Could you check a few things on this model? Use its own coordinates, in mm. A direction names the side the tool comes from. Coordinates: 2 decimals unless noted, no trailing zeros. Loops run counter-clockwise (first coordinate to the right, second up) from the corner with the lowest first, then second, coordinate; pieces in that order, holes last.
from build123d import *

# Parameters (mm, degrees)
SKIZZE2_R                       = 1.825
SKIZZE2_R_2                     = 2.9
AUFSATZ_LINEAR_AUSTRAGEN1_DEPTH = 10
SCHNITT_LINEAR_START            = -2.75
SCHNITT_LINEAR_AUSTRAGEN1_DEPTH = 2.75
VERRUNDUNG1_R                   = 10
VERRUNDUNG2_R                   = 10
AUFSATZ_LINEAR_START            = -7.25
SKIZZE5_R                       = 9
SKIZZE5_R_2                     = 5
AUFSATZ_LINEAR_AUSTRAGEN2_DEPTH = 7.25
AUFSATZ_LINEAR_AUSTRAGEN3_DEPTH = 7.25
KREISMUSTER1_COUNT              = 20
SCHNITT_LINEAR_AUSTRAGEN3_DEPTH = 39.948684188


with BuildPart() as part:
    # Skizze2 → Aufsatz-Linear austragen1 (new body)
    with BuildSketch(Plane(origin=(0, 0, 0), x_dir=(1, 0, 0), z_dir=(0, 1, 0))):
        with BuildLine():
            Line((-25, 5), (25, 5))
            ThreePointArc((25, 5), (30, 0), (25, -5))
            Line((25, -5), (-25, -5))
            ThreePointArc((-25, -5), (-30, 0), (-25, 5))
        make_face()
        with Locations(Location((-25, 0, 0), (0, 0, 270))):
            Circle(SKIZZE2_R, mode=Mode.SUBTRACT)
        with Locations(Location((25, 0, 0), (0, 0, 270))):
            Circle(SKIZZE2_R_2, mode=Mode.SUBTRACT)
    extrude(amount=AUFSATZ_LINEAR_AUSTRAGEN1_DEPTH)

    # Skizze4 → Schnitt-Linear austragen1 (cut)
    with BuildSketch(Plane(origin=(0, 10, 0), x_dir=(1, 0, 0), z_dir=(0, 1, 0)).offset(SCHNITT_LINEAR_START)):
        with BuildLine():
            Line((25, 5), (0, 5))
            Line((0, 5), (0, -5))
            Line((0, -5), (25, -5))
            ThreePointArc((25, -5), (30, 0), (25, 5))
        make_face()
    extrude(amount=SCHNITT_LINEAR_AUSTRAGEN1_DEPTH, mode=Mode.SUBTRACT)

    # Verrundung1
    # the kernel refuses this fillet: 10 mm, written as the material it adds along each edge
    with BuildSketch(Plane(origin=(0, 7.25, -5), x_dir=(1, 0, 0), z_dir=(0, 0, 1))) as verrundung1_piece_1:
        with BuildLine():
            CenterArc((6.887488657, 10), VERRUNDUNG1_R, 226.468847833, 43.531152167)
            Line((0, 2.75), (-0.137749773, 2.605))
            ThreePointArc((-0.137749773, 2.605), (-0.2, 1.375), (-0.2, 0))
            Line((-0.2, 0), (0, -0.2))
            Line((0, -0.2), (6.887488657, -0.2))
            Line((6.887488657, -0.2), (6.887488657, 0))
        make_face()
    extrude(amount=10)

    # Verrundung2
    verrundung2_edges = [part.edges().sort_by_distance(p)[0] for p in [
        (0, 10, 0),
    ]]
    fillet(verrundung2_edges, radius=VERRUNDUNG2_R)

    # Skizze5 → Aufsatz-Linear austragen2 (add)
    with BuildSketch(Plane(origin=(0, 7.25, 0), x_dir=(1, 0, 0), z_dir=(0, 1, 0)).offset(AUFSATZ_LINEAR_START)):
        with Locations((25, 0)):
            Circle(SKIZZE5_R)
        with Locations((25, 0)):
            Circle(SKIZZE5_R_2, mode=Mode.SUBTRACT)
    extrude(amount=AUFSATZ_LINEAR_AUSTRAGEN2_DEPTH)

    # Skizze6 → Aufsatz-Linear austragen3 (add)
    with BuildSketch(Plane(origin=(0, 7.25, 0), x_dir=(1, 0, 0), z_dir=(0, 1, 0)).offset(AUFSATZ_LINEAR_START)):
        with BuildLine():
            Line((36, -0.35), (36, 0.35))
            ThreePointArc((36, 0.35), (34.995800842, 0.693259833), (33.954886934, 0.9))
            ThreePointArc((33.954886934, 0.9), (34, 0), (33.954886934, -0.9))
            ThreePointArc((33.954886934, -0.9), (34.995800842, -0.693259833), (36, -0.35))
        make_face()
    aufsatz_linear_austragen3 = extrude(amount=AUFSATZ_LINEAR_AUSTRAGEN3_DEPTH)

    # Kreismuster1: Aufsatz-Linear austragen3 ×20 about axis
    kreismuster1_axis = Axis((25, 0, 0), (0, 1, 0))
    for i in range(1, KREISMUSTER1_COUNT):
        add(aufsatz_linear_austragen3.rotate(kreismuster1_axis, i * 360 / KREISMUSTER1_COUNT))

    # Skizze9 → Schnitt-Linear austragen3 (cut, through all)
    with BuildSketch(Plane.XZ):
        with BuildLine():
            Line((-11, 3), (11, 3))
            ThreePointArc((11, 3), (14, 0), (11, -3))
            Line((11, -3), (-11, -3))
            ThreePointArc((-11, -3), (-14, 0), (-11, 3))
        make_face()
    extrude(amount=-SCHNITT_LINEAR_AUSTRAGEN3_DEPTH, mode=Mode.SUBTRACT)


solid = part.part
(1) I need wall thicknesses on probe 1 along X at (y, z) = (3, 0) (3 decimals); probe 2 along Z at (x, y) = (-6, 2.5); probe 3 along Z at (x, y) = (25, 2.75). Which ranges of each line are inside material? Lowest first, please.
Answers:
probe 1: x = -30 to -26.825, -23.175 to -14, 14 to 22.1, 27.9 to 36
probe 2: z = -5 to -3, 3 to 5
probe 3: z = -11 to -2.9, 2.9 to 11
(2) Imagine slicing it at B-B, the plane x = -13. Write out the boundary of the cut face in (y, z), and give its area (3 significant figures).
Answers:
outline: (0, -5) - (10, -5) - (10, -2.24) - (0, -2.24) - close; (0, 2.24) - (10, 2.24) - (10, 5) - (0, 5) - close
area: 55.3 mm2
(3) Imagine slicing it at D-D, the plane x = 13. Write out the boundary of the cut face in (y, z).
Answers:
outline: (0, -5) - (7.25, -5) - (7.25, -2.24) - (0, -2.24) - close; (0, 2.24) - (7.25, 2.24) - (7.25, 5) - (0, 5) - close
(4) Imagine slicing it at C-C, the plane y = 5.5. State how many separate pieces and enclosed holes the cut face has, and give its area (3 significant figures).
Answers:
separate pieces: 1
enclosed holes: 3
area: 557 mm2
(5) For pin 1 (2 mm diameter, centred on y = 6, z = -7, fed in from +X); pin 2 (2 mm diameter, centred on y = 4.5, z = -4.5, fed in from -X); pin 3 (3 mm diameter, centred on x = 9.5, y = 8.5, fed in from +Z); pin 4 (3.5 mm diameter, centred on x = 25, z = 0, fed in from +Y), each with a flat end and sliding along its axis, tell me the tip position at first contact or that it passes through.
Answers:
pin 1: stops at x = 34.1
pin 2: stops at x = -28.57
pin 3: stops at z = 5
pin 4: passes through
(6) We'd pull the mould along X, two halves only. Please class faces 6 (the face through (-30, 5, 0)), 7 (the face through (-26.78, 4.93, -0.4)), 8 (the face through (35.01, 3.57, -0.69)): +X half, -X half, draft (parallel to the pull), parting line (faces both ways), or undercut.
Answers:
face 6: -X half
face 7: undercut
face 8: +X half
(7) Which directions (+Z, -Z, +X, -X, +Y, -Y) give clear straight access to the entire face, cutting with the end or side of a thin tool? Please do faces 1 (the face through (25.697, 3.574, -9.981)), 2 (the face through (27.421, 3.574, 9.708)), 3 (the face through (9, 0, 4)), 4 (the face through (34.733, 3.574, 2.438)), 5 (the face through (28.747, 3.574, -9.277)).
Answers:
face 1: -Z, +Y, -Y
face 2: +Z, +Y, -Y
face 3: +Z, -Z, +X, -X, -Y
face 4: +X, +Y, -Y
face 5: +Y, -Y
(8) Imagine slicing it at A-A, the plane z = 9.75. Write out the boundary of the cut face in (x, y).
Answers:
outline: (21.24, 0) - (22.55, 0) - (22.55, 7.25) - (21.24, 7.25) - close; (24.24, 0) - (25.76, 0) - (25.76, 7.25) - (24.24, 7.25) - close; (27.45, 0) - (28.76, 0) - (28.76, 7.25) - (27.45, 7.25) - close
